Here's how the part is built. I have some questions about the finished solid (model axes, mm). A direction names the side the tool comes from. Round coordinates to 2 decimals unless told otherwise and drop trailing zeros. Write each loop counter-clockwise with the first axis right and the second up, starting at its lowest first coordinate (ties: lowest second). Pieces come first, ordered by that corner, then holes. Notation, with made-up numbers: (-35.5, 86.25) - (2.5, 86.25) arc R23 ccw to (2.5, 113.25) - close; hole circle Ø7 at (28, 80). An arc over 180 degrees is marked (long way). One line per item, written item: value. Start each with the question number.
Item 1: For faces 5 (the face through (51.65, 0.04, 1.48)), 6 (the face through (-1, 2, 3)), which set-ups out of +Z, -Z, +X, -X, +Y, -Y let a thin tool reach every point of the face, with its end or its side?
Item 2: Imagine slicing it at A-A, the plane z = 2.25. Please give me the cut outline in (x, y).
Item 3: Imagine slicing it at B-B, the plane x = 35. Please give me the cut outline in (y, z).
Item 4: If I drill on line 1 (Y direction, x = 30.5, z = 1.4); line 2 (X direction, y = -0.25, z = 0.2); line 3 (X direction, y = -1.5, z = 2.25), over which ranges is the centre line in solid material (lowest first)?
Item 5: Thinking about a two-plate mould opening in Y: for faces 1 (the face through (54.4, -2.93, 1.52)), 2 (the face through (54.4, 2.93, 1.52)), 3 (the face through (1, -1.65, 1)), 4 (the face through (-51.65, -0.04, 1.48)), which applies, released by +Y, released by -Y, zero draft, split by the parting line, or undercut?
Item 6: Imagine slicing it at C-C, the plane y = -0.5. Please give me the cut outline in (x, z), then the cut area to 3 significant figures.
```python
from build123d import *

# Parameters (mm, degrees)
SKETCH_1_W      = 110
SKETCH_1_H      = 7
EXTRUDE_1_DEPTH = 3
FILLET_1_R      = 2


with BuildPart() as part:
    # 草图1 → 凸台-拉伸1 (new body)
    with BuildSketch(Plane.XY):
        Rectangle(SKETCH_1_W, SKETCH_1_H)
        with BuildLine():
            Line((-50, 1.65), (50, 1.65))
            ThreePointArc((50, 1.65), (51.65, 0), (50, -1.65))
            Line((50, -1.65), (-50, -1.65))
            ThreePointArc((-50, -1.65), (-51.65, 0), (-50, 1.65))
        make_face(mode=Mode.SUBTRACT)
    extrude(amount=EXTRUDE_1_DEPTH)

    # 圆角1
    fillet_1_edges = [part.edges().sort_by_distance(p)[0] for p in [
        (55, -3.5, 1.5),
        (-55, -3.5, 1.5),
        (-55, 3.5, 1.5),
        (55, 3.5, 1.5),
    ]]
    fillet(fillet_1_edges, radius=FILLET_1_R)


solid = part.part
```
Values follow:
1. face 5: +Z, -Z
1. face 6: +Z, +X, -X, +Y, -Y
2. outline: (-55, -1.5) arc R2 ccw to (-53, -3.5) - (53, -3.5) arc R2 ccw to (55, -1.5) - (55, 1.5) arc R2 ccw to (53, 3.5) - (-53, 3.5) arc R2 ccw to (-55, 1.5) - close; hole (-50, -1.65) - (50, -1.65) arc R1.65 ccw to (50, 1.65) - (-50, 1.65) arc R1.65 ccw to start
3. outline: (-3.5, 0) - (-1.65, 0) - (-1.65, 3) - (-3.5, 3) - close; (1.65, 0) - (3.5, 0) - (3.5, 3) - (1.65, 3) - close
4. line 1: y = -3.5 to -1.65, 1.65 to 3.5
4. line 2: x = -55 to -51.63, 51.63 to 55
4. line 3: x = -55 to -50.69, 50.69 to 55
5. face 1: released by -Y
5. face 2: released by +Y
5. face 3: undercut
5. face 4: undercut
6. outline: (-55, 0) - (-51.57, 0) - (-51.57, 3) - (-55, 3) - close; (51.57, 0) - (55, 0) - (55, 3) - (51.57, 3) - close
6. area: 20.6 mm^2
